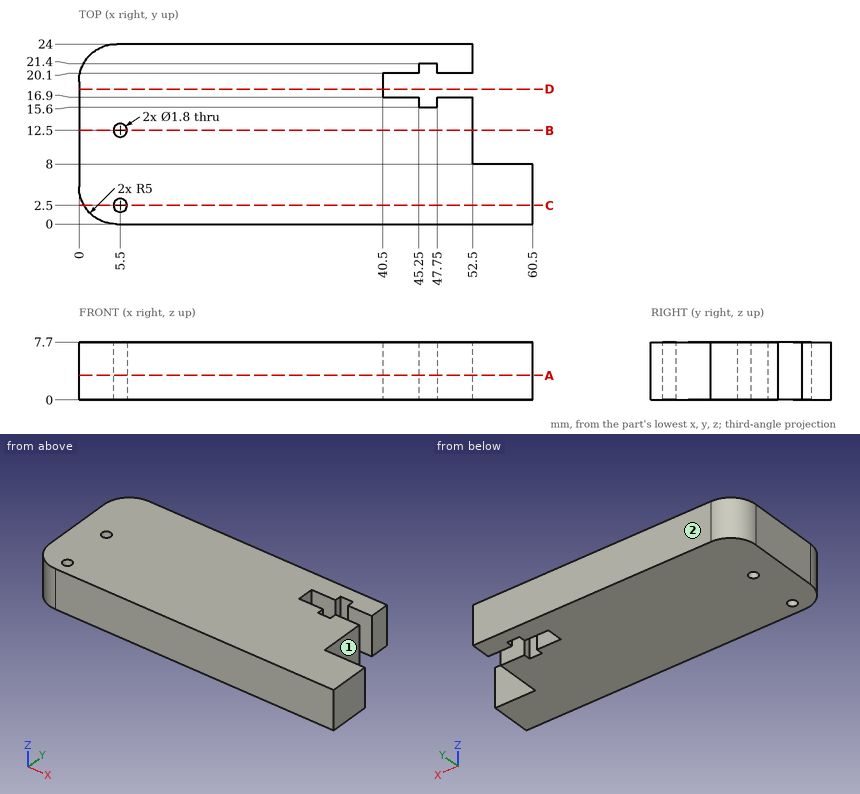
Job drawing, mm, ordinate dimensions from the low corner. One solid piece. A direction names the side the tool comes from. Give positions to 0.01 mm unless a question says otherwise; leave off trailing zeros. Write each loop counter-clockwise with the first axis right and the second up, starting at its lowest first coordinate (ties: lowest second). Pieces come first, ordered by that corner, then holes. Notation, with made-up numbers: (16.25, 77.25) - (26.25, 77.25) arc R27 ccw to (26.25, 103.25) - close; hole circle Ø7 at (82, 8.5). An arc over 180 degrees is marked (long way). Answer as CSV lines item,"result".
1. Pin check, flat tips, straight feed: pin 1 (2.5 mm diameter, centred on x = 56.5, z = 5.5, fed in from +Y); pin 2 (1.2 mm diameter, centred on y = 22, z = 5, fed in from +X); pin 3 (1.6 mm diameter, centred on y = 18, z = 4.5, fed in from +X). Stop position of each tip, or through.
Responses:
pin 1,"stops at y = 8"
pin 2,"stops at x = 52.5"
pin 3,"stops at x = 40.5"
2. Band-saw the part on A-A (z = 3.25). Write the cut outline in (x, y).
Responses:
outline,"(0, 5) arc R5 ccw to (5, 0) - (60.5, 0) - (60.5, 8) - (52.5, 8) - (52.5, 16.9) - (47.75, 16.9) - (47.75, 15.6) - (45.25, 15.6) - (45.25, 16.9) - (40.5, 16.9) - (40.5, 20.1) - (45.25, 20.1) - (45.25, 21.4) - (47.75, 21.4) - (47.75, 20.1) - (52.5, 20.1) - (52.5, 24) - (5, 24) arc R5 ccw to (0, 19) - close; hole circle Ø1.8 at (5.5, 2.5); hole circle Ø1.8 at (5.5, 12.5)"
3. Band-saw the part on B-B (y = 12.5). Write the cut outline in (x, z), and give its area (3 significant figures).
Responses:
outline,"(0, 0) - (4.6, 0) - (4.6, 7.7) - (0, 7.7) - close; (6.4, 0) - (52.5, 0) - (52.5, 7.7) - (6.4, 7.7) - close"
area,"390 mm2"
4. 3-axis set-ups, long thin cutter, end or side, ignore diameter. For the marked faces 1 and 2: which of +Z, -Z, +X, -X, +Y, -Y reach the whole face in a straight line?
Responses:
face 1,"+Z, -Z, +X, +Y"
face 2,"+Z, -Z, +X, -X, +Y"
5. Band-saw the part on D-D (y = 18). Write the cut outline in (x, z), and give its area (3 significant figures).
Responses:
outline,"(0, 0) - (40.5, 0) - (40.5, 7.7) - (0, 7.7) - close"
area,"312 mm2"
6. Drill centre lines: L1, parallel to Y at x = 5.5, z = 3.25; L2, parallel to Y at x = 45, z = 6.75; L3, parallel to Y at x = 46, z = 2. Where is each one in solid material? Low to high. Write a range as [from, to].
Responses:
L1,"y = [0, 1.6], [3.4, 11.6], [13.4, 24]"
L2,"y = [0, 16.9], [20.1, 24]"
L3,"y = [0, 15.6], [21.4, 24]"
7. Band-saw the part on C-C (y = 2.5). Write the cut outline in (x, z), and give its area (3 significant figures).
Responses:
outline,"(0.67, 0) - (4.6, 0) - (4.6, 7.7) - (0.67, 7.7) - close; (6.4, 0) - (60.5, 0) - (60.5, 7.7) - (6.4, 7.7) - close"
area,"447 mm2"
